from build123d import *

# Parameters (mm, degrees)
F0_R      = 25.4
F1_DEPTH  = 25.4
F2_R      = 5.08
F1_FACE_R = 20.32
F3_DEPTH  = 17.018


with BuildPart() as f1:
    # F0 (on Front) → F1 (new body)
    with BuildSketch(Plane.XZ):
        Circle(F0_R)
    extrude(amount=F1_DEPTH)

    # F2
    f2_edges = [f1.edges().sort_by_distance(p)[0] for p in [
        (25.4, -12.7, 0),
        (-25.4, 0, 0),
        (-25.4, -25.4, 0),
    ]]
    fillet(f2_edges, radius=F2_R)

    # F1_face (on face) → F3 (cut)
    with BuildSketch(Plane.XZ.offset(25.4)):
        Circle(F1_FACE_R)
    extrude(amount=-F3_DEPTH, mode=Mode.SUBTRACT)


solid = f1.part
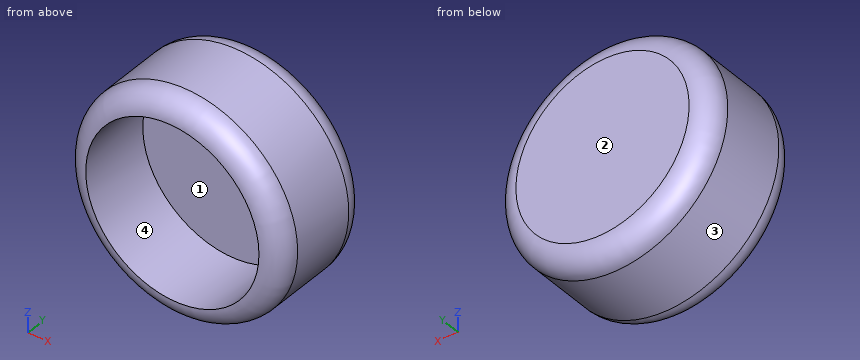
Input: part model. Units: mm. Frame: model coordinates. Face numbers are marked on the shaded views. Coordinates: 2 decimals unless noted, no trailing zeros. Loops run counter-clockwise (first coordinate to the right, second up) from the corner with the lowest first, then second, coordinate; pieces in that order, holes last. Notation, with made-up numbers: (2.5, -26.75) -> (47.5, -26.75) arc R18 ccw to (47.5, 1.25) -> close; hole circle Ø3 at (-12.75, 13.25). An arc over 180 degrees is marked (long way). One line per item, written item: value.
(1) Cut plane A-A (x = 0). Output: boundary loops of the cut face in (y, z), then the cut area to 3 significant figures.
Answer below:
outline: (-25.4, -20.32) arc R5.08 ccw to (-20.32, -25.4) -> (-5.08, -25.4) arc R5.08 ccw to (0, -20.32) -> (0, 20.32) arc R5.08 ccw to (-5.08, 25.4) -> (-20.32, 25.4) arc R5.08 ccw to (-25.4, 20.32) -> (-8.38, 20.32) -> (-8.38, -20.32) -> close
area: 577 mm2
(2) Cut plane B-B (z = 0). Output: boundary loops of the cut face in (x, y), then the cut area to 3 significant figures.
Answer below:
outline: (-25.4, -20.32) arc R5.08 ccw to (-20.32, -25.4) -> (-20.32, -8.38) -> (20.32, -8.38) -> (20.32, -25.4) arc R5.08 ccw to (25.4, -20.32) -> (25.4, -5.08) arc R5.08 ccw to (20.32, 0) -> (-20.32, 0) arc R5.08 ccw to (-25.4, -5.08) -> close
area: 577 mm2
(3) Ray query, line 1 along Z through (x, y) = (0, -13.75); line 2 along Y through (x, z) = (2.5, 12); line 3 along Z through (x, y) = (4, -11.5). Return the intervals inside material, ascending.
Answer below:
line 1: z = -25.4 to -20.32, 20.32 to 25.4
line 2: y = -8.38 to 0
line 3: z = -25.08 to -19.92, 19.92 to 25.08
(4) Draft query along Z for the marked faces 1, 2, 3 and 4. Return one class per face: pulls with the +Z half, pulls with the -Z half, needs draft (parallel to the pull), parting line crosses it, or undercut.
Answer below:
face 1: undercut
face 2: needs draft
face 3: parting line crosses it
face 4: undercut
(5) Pin query (flat end, axial travel): pin 1 Ø1.5 at (y, z) = (-22, 14) entering from +X; pin 2 Ø6 at (y, z) = (-7, -3) entering from -X; pin 3 Ø1.5 at (y, z) = (-18, 6.5) entering from -X; pin 4 Ø1 at (y, z) = (-5.5, 13) entering from +X. Return the tip coordinate at first contact, or that it passes through.
Answer below:
pin 1: stops at x = 21.41
pin 2: stops at x = -25.4
pin 3: stops at x = -24.74
pin 4: stops at x = 22.11
